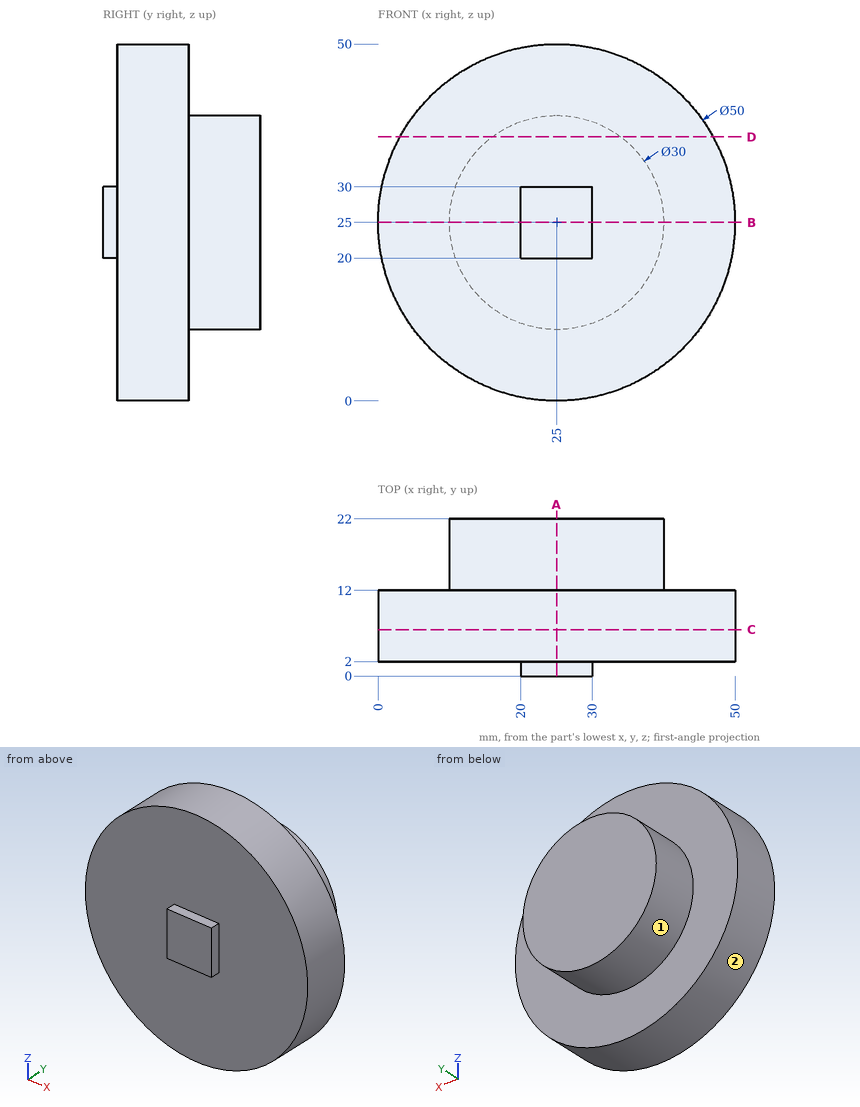
Input: dimensioned drawing with shaded views. Units: mm. Origin: part minimum x, y, z. A direction names the side the tool comes from. Give positions to 0.01 mm unless a question says otherwise; leave off trailing zeros. Loops run counter-clockwise (first coordinate to the right, second up) from the corner with the lowest first, then second, coordinate; pieces in that order, holes last. Notation, with made-up numbers: M 40.25,24 L 58.25,24 A8 cw 58.25,35 Z; hole C 6,75.5 d4. An arc over 180 degrees is marked long. Put each result on its own line as item: value. Start each with the question number.
1) Cut plane D-D (z = 37). Output: boundary loops of the cut face in (x, y).
2) Cut plane C-C (y = 6.5). Output: boundary loops of the cut face in (x, z).
3) Cut plane B-B (z = 25). Output: boundary loops of the cut face in (x, y).
4) Ray query, line 1 along Y through (x, z) = (6.5, 21.5); line 2 along Y through (x, z) = (17, 33); line 3 along X through (y, z) = (3.5, 37). Return the intervals inside material, ascending.
5) Cut plane A-A (x = 25). Output: boundary loops of the cut face in (y, z).
6) Contact query for flat-ended pins moving along their axis: pin 1 (2 mm diameter, centred on x = 39.5, y = 9.5, fed in from +Z); pin 2 (15 mm diameter, centred on x = 25.5, z = 29.5, fed in from -Y); pin 3 (4 mm diameter, centred on y = 12, z = 26, fed in from +X); pin 4 (2 mm diameter, centred on y = 0.5, z = 23, fed in from +X). Output: stop coordinate, or through.
7) Access query for the marked faces 1 and 2. Directions: +Z, -Z, +X, -X, +Y, -Y. A direction counts if a zero-diameter tool reaches every point of the face in a straight line with its end or side. Return the directions, or none.
Verdict:
1. outline: M 3.07,2 L 46.93,2 L 46.93,12 L 34,12 L 34,22 L 16,22 L 16,12 L 3.07,12 Z
2. outline: C 25,25 d50
3. outline: M 0,2 L 20,2 L 20,0 L 30,0 L 30,2 L 50,2 L 50,12 L 40,12 L 40,22 L 10,22 L 10,12 L 0,12 Z
4. line 1: 2 to 12
4. line 2: 2 to 22
4. line 3: 3.07 to 46.93
5. outline: M 0,20 L 2,20 L 2,0 L 12,0 L 12,10 L 22,10 L 22,40 L 12,40 L 12,50 L 2,50 L 2,30 L 0,30 Z
6. pin 1: z = 46.04
6. pin 2: y = 0
6. pin 3: x = 50
6. pin 4: x = 30
7. face 1: +Y
7. face 2: +Y, -Y
